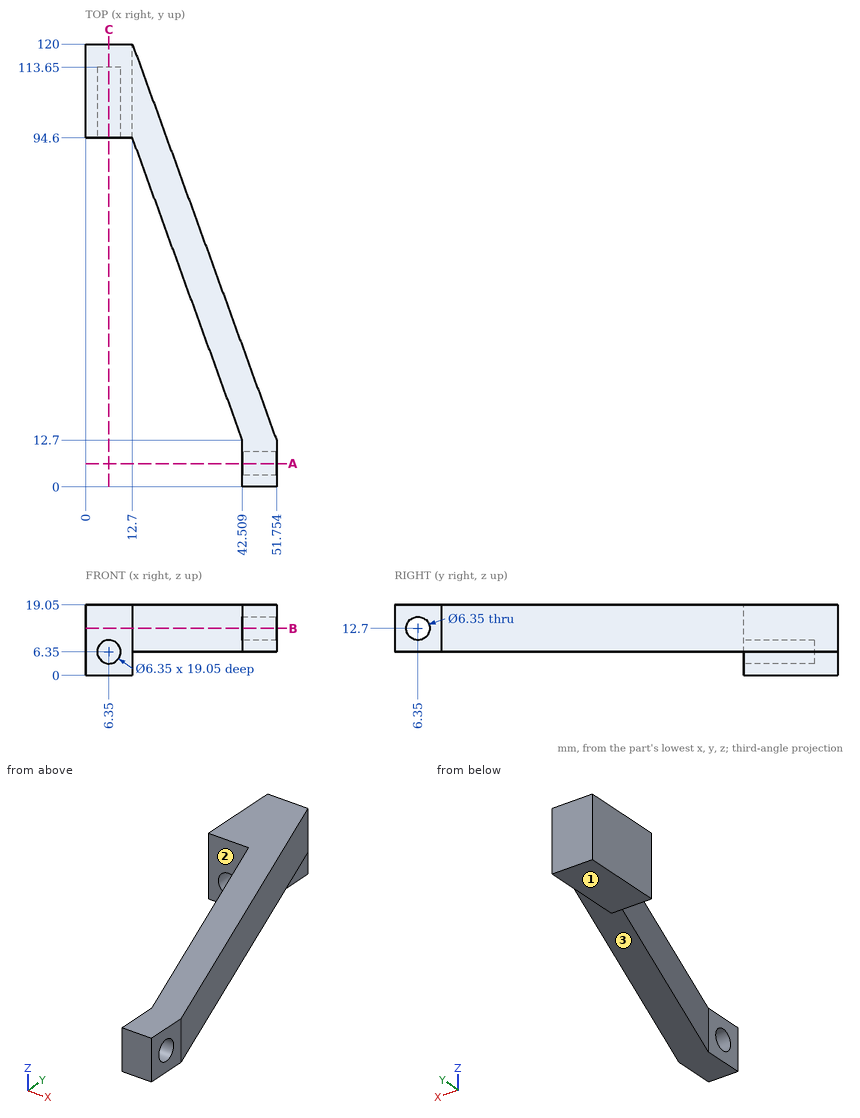
Source: three-view drawing plus pictorial views. Frame: mm from the lowest corner of the part. A direction names the side the tool comes from. Give positions to 0.01 mm unless a question says otherwise; leave off trailing zeros. Order: outer loops, then holes, each group sorted by start corner. A loop starts at its lowest first (then second) coordinate and runs counter-clockwise, first axis right, second up. Notation, with made-up numbers: (-23.75, -26) -> (18.25, -26) arc R37 ccw to (18.25, 13) -> close; hole circle Ø1 at (-4.75, 58). An arc over 180 degrees is marked (long way). Write each question's results on one line, items separated by ' | '. Start each with the question number.
Item 1: Contact query for flat-ended pins moving along their axis: P1, Ø10, axis at y = 42, z = 8.5, coming from the +X side; P2, Ø7.5, axis at y = 6.35, z = 12.7, coming from the +X side; P3, Ø6.5, axis at y = 3.5, z = 11, coming from the -X side; P4, Ø4, axis at x = 8, z = 5, coming from the -Y side. Output: stop coordinate, or through.
Item 2: Cut plane A-A on y = 6.35. Return the cut outline in (x, z) (3 decimals), then the cut area to 3 significant figures.
Item 3: Line query: line 1 (Z direction, x = 6.35, y = 100.25) (3 decimals); line 2 (Z direction, x = 45, y = 6); line 3 (Y direction, x = 7, z = 6). Output: solid intervals per line, ascending.
Item 4: Set-up query: the marked faces 1, 2 and 3. Return all of +Z, -Z, +X, -X, +Y, -Y with unobstructed straight access to the full face (end or side cutting, diameter ignored); none if empty.
Item 5: Cut plane B-B on z = 12.7. Return the cut outline in (x, y) (3 decimals), then the cut area to 3 significant figures.
Item 6: Cut plane C-C on x = 6.35. Return the cut outline in (y, z) (3 decimals), then the cut area to 3 significant figures.
Established:
1) P1: x = 42.91 | P2: x = 51.75 | P3: x = 42.51 | P4: y = 94.6
2) outline: (42.509, 6.35) -> (51.754, 6.35) -> (51.754, 9.525) -> (42.509, 9.525) -> close; (42.509, 15.875) -> (51.754, 15.875) -> (51.754, 19.05) -> (42.509, 19.05) -> close | area: 58.7 mm^2
3) line 1: 0 to 3.175, 9.525 to 19.05 | line 2: 6.35 to 9.54, 15.86 to 19.05 | line 3: 113.65 to 120
4) face 1: -Z, +X, -X, +Y, -Y | face 2: +Z, -Z, -X, -Y | face 3: -Z, +X, +Y, -Y
5) outline: (0, 94.6) -> (12.7, 94.6) -> (42.509, 12.7) -> (42.509, 9.525) -> (51.754, 9.525) -> (51.754, 12.7) -> (12.7, 120) -> (0, 120) -> close; (42.509, 0) -> (51.754, 0) -> (51.754, 3.175) -> (42.509, 3.175) -> close | area: 1,260 mm^2
6) outline: (94.6, 0) -> (120, 0) -> (120, 19.05) -> (94.6, 19.05) -> (94.6, 9.525) -> (113.65, 9.525) -> (113.65, 3.175) -> (94.6, 3.175) -> close | area: 363 mm^2
